Design review of the part built by this model. Coordinates are the model's own, in mm. Give positions to 0.01 mm unless a question says otherwise; leave off trailing zeros. Write each loop counter-clockwise with the first axis right and the second up, starting at its lowest first coordinate (ties: lowest second). Pieces come first, ordered by that corner, then holes. Notation, with made-up numbers: (-15.5, 78.25) -> (-1.5, 78.25) arc R20 cw to (-1.5, 117.25) -> close; hole circle Ø9 at (61.25, 75). An arc over 180 degrees is marked (long way). Answer as a JSON object with one key per item and string values.
```python
from build123d import *

# Parameters (mm, degrees)
F0_R        = 62.874462
F0_R_2      = 9.295278
F1_DEPTH    = 9.652
F1_FACE_R   = 62.874462
F1_FACE_R_2 = 9.295278
F2_DEPTH    = 25.4


with BuildPart() as f1:
    # F0 (on Top) → F1 (new body)
    with BuildSketch(Plane.XY):
        Circle(F0_R)
        with Locations((-16.614098, -43.2841)):
            Circle(F0_R_2, mode=Mode.SUBTRACT)
        with Locations((-42.354422, -18.858539)):
            Circle(F0_R_2, mode=Mode.SUBTRACT)
        with Locations((18.858539, -42.354422)):
            Circle(F0_R_2, mode=Mode.SUBTRACT)
        with Locations((43.2841, -16.614098)):
            Circle(F0_R_2, mode=Mode.SUBTRACT)
        with Locations((-43.2841, 16.614098)):
            Circle(F0_R_2, mode=Mode.SUBTRACT)
        with Locations((-18.858539, 42.354422)):
            Circle(F0_R_2, mode=Mode.SUBTRACT)
        with Locations((42.354422, 18.858539)):
            Circle(F0_R_2, mode=Mode.SUBTRACT)
        with Locations((16.614098, 43.2841)):
            Circle(F0_R_2, mode=Mode.SUBTRACT)
    extrude(amount=F1_DEPTH)

    # F1_face (on face) → F2 (join)
    with BuildSketch(Plane.XY.offset(9.652)):
        Circle(F1_FACE_R)
        with Locations((-16.614098, -43.2841)):
            Circle(F1_FACE_R_2, mode=Mode.SUBTRACT)
        with Locations((-42.354422, -18.858539)):
            Circle(F1_FACE_R_2, mode=Mode.SUBTRACT)
        with Locations((18.858539, -42.354422)):
            Circle(F1_FACE_R_2, mode=Mode.SUBTRACT)
        with Locations((43.2841, -16.614098)):
            Circle(F1_FACE_R_2, mode=Mode.SUBTRACT)
        with Locations((-43.2841, 16.614098)):
            Circle(F1_FACE_R_2, mode=Mode.SUBTRACT)
        with Locations((-18.858539, 42.354422)):
            Circle(F1_FACE_R_2, mode=Mode.SUBTRACT)
        with Locations((42.354422, 18.858539)):
            Circle(F1_FACE_R_2, mode=Mode.SUBTRACT)
        with Locations((16.614098, 43.2841)):
            Circle(F1_FACE_R_2, mode=Mode.SUBTRACT)
    extrude(amount=F2_DEPTH)


solid = f1.part
```
(1) The part is to be moulded in two halves that separate along Y. For faces 1 (the flat face through (-1, 1, 35.052)), 2 (the cylindrical face through (40.339, 9.784, 17.281)), 3 (the cylindrical face through (-49.895, -38.258, 17.281)), 4 (the cylindrical face through (14.6, 34.21, 17.28)), say which applies: +Y half, -Y half, draft (parallel to the pull), parting line (faces both ways), or undercut.
Here are the results:
{"face 1": "draft", "face 2": "undercut", "face 3": "parting line", "face 4": "undercut"}
(2) We need section B-B, the plane x = -47.5. State the section outline as (y, z) points.
Here are the results:
{"outline": "(-41.19, 0) -> (-26.6, 0) -> (-26.6, 35.05) -> (-41.19, 35.05) -> close; (-11.12, 0) -> (8.33, 0) -> (8.33, 35.05) -> (-11.12, 35.05) -> close; (24.9, 0) -> (41.19, 0) -> (41.19, 35.05) -> (24.9, 35.05) -> close"}
(3) We need section C-C, the plane z = 25.5. Give the number of separate pieces and of enclosed holes in the cut face, then the cut area to 3 significant figures.
Here are the results:
{"separate pieces": "1", "enclosed holes": "8", "area": "10,200 mm²"}
(4) Clearance check with flat-ended pins moving along their axes: pin 1 (6 mm diameter, centred on x = -22, z = 25, fed in from -Y); pin 2 (1 mm diameter, centred on y = -44.5, z = 31, fed in from +X); pin 3 (1 mm diameter, centred on x = 0.5, z = 25.5, fed in from -Y). State where each tip first meets the part, or that it passes through.
Here are the results:
{"pin 1": "stops at y = -59.93", "pin 2": "stops at x = 44.91", "pin 3": "stops at y = -62.87"}
(5) For line 1 along X through (y, z) = (-48.5, 17); line 2 along Y through (x, z) = (41, 19.5); line 3 along X through (y, z) = (11, 10), list the stretches that pass through material, from the lowest coordinate up.
Here are the results:
{"line 1": "x = -40.01 to -24.31, -8.92 to 11.88, 25.83 to 40.01", "line 2": "y = -47.67 to -25.62, -7.6 to 9.66, 28.05 to 47.67", "line 3": "x = -61.9 to -50.69, -35.88 to 37.39, 47.32 to 61.9"}
(6) We need section A-A, the plane y = -22. State the section outline as (x, z) points, then the cut area to 3 significant figures.
Here are the results:
{"outline": "(-58.9, 0) -> (-51.1, 0) -> (-51.1, 35.05) -> (-58.9, 35.05) -> close; (-33.61, 0) -> (35.71, 0) -> (35.71, 35.05) -> (-33.61, 35.05) -> close; (50.86, 0) -> (58.9, 0) -> (58.9, 35.05) -> (50.86, 35.05) -> close", "area": "2,980 mm²"}
